Design review of the part built by this model. Coordinates are the model's own, in mm. A direction names the side the tool comes from. Coordinates: 2 decimals unless noted, no trailing zeros. Write each loop counter-clockwise with the first axis right and the second up, starting at its lowest first coordinate (ties: lowest second). Pieces come first, ordered by that corner, then holes.
Q1. Mouldability with a two-part tool opening along Z and no side actions: class faces 1 (the flat face through (6.324, 7.395, -27.347)), 2 (the flat face through (-5.32, 32.96, 32.43)), 3 (the flat face through (-9, 7, -16)), 4 (the cylindrical face through (-16.545, 7.395, -0.389)) as pulls with the +Z half, pulls with the -Z half, needs draft (parallel to the pull), parting line crosses it, or undercut.
Q2. Take a section at C-C (z = -9). Give the boundary of the cut face in (x, y).
Q3. Take a section at D-D (z = 26). Give the boundary of the cut face in (x, y).
Q4. Insertion check: pin 1 (4 mm diameter, centred on y = 6, z = -16.5, fed in from +X); pin 2 (3 mm diameter, centred on y = 27, z = 35.5, fed in from -X); pin 3 (1.2 mm diameter, centred on x = -7.5, y = 33, fed in from -Z); pin 4 (1.5 mm diameter, centred on x = -10, z = 10, fed in from -Y). Each pin has a flat end and moves straight along its axis. Give the tip position at first contact, or say it passes through.
Q5. For probe 1 along Z at (x, y) = (9.5, 4.5); probe 2 along Z at (x, y) = (-9.5, 22); probe 3 along Z at (x, y) = (8, 16.5), list the stretches that pass through material, from the lowest coordinate up.
Q6. Machinability: for faces 5 (the flat face through (9, 33, 31.469)), 6 (the flat face through (5, 7, -17.756)), 7 (the flat face through (10, 32, 35)), 8 (the flat face through (-10, 25, 20)), 9 (the flat face through (-9, 33, 31.469)), which of the approach directions +Z, -Z, +X, -X, +Y, -Y give a long, thin tool a straight path to every point of the face, cutting with its end or side? Answer none if there is none.
Q7. Take a section at B-B (y = 28.5). Give the boundary of the cut face in (x, z), and give its area (3 significant figures).
Q8. Take a section at A-A (x = -11.5). Give the boundary of the cut face in (y, z), and give its area (3 significant figures).
Autodesk Inventor part; units mm, degrees
ref_plane "YZ Plane" through (0, 0, 0) normal (1, 0, 0) x (0, 1, 0)
ref_plane "XZ Plane" through (0, 0, 0) normal (0, 1, 0) x (-1, 0, 0)
ref_plane "XY Plane" through (0, 0, 0) normal (0, 0, 1) x (1, 0, 0)
sketch "스케치1" plane through (0, 0, 0) normal (0, 1, 0) x (-1, 0, 0)
  arc A0 (0, -14.55) -> (-2.5266, -14.329) centre (0, 0) ccw
  line L0 (-2.5656, -14.55) -> (-7, -14.55)
  line L1 (7, -14.55) -> (7, -12.7555)
  line L2 (-7, -14.55) -> (-7, -12.7555)
  arc A1 (2.8739, -16.2986) -> (-2.8739, -16.2986) centre (0, 0) ccw
  line L3 (7, -12.7555) -> (7, -17.7555)
  line L4 (-7, -12.7555) -> (-7, -17.7555)
  line L5 (-7, -17.7555) -> (-9, -17.7555)
  line L6 (-9, -17.7555) -> (-9, -13.8889)
  line L7 (7, -17.7555) -> (9, -17.7555)
  line L8 (9, -17.7555) -> (9, -13.8889)
  line L9 (0, 0) -> (23.7529, 0) construction
  line L10 (0, 0) -> (23.7529, 0) construction
  line L11 (4.1247, -23.3921) -> (7.0791, -22.8711)
  line L12 (7.0791, -22.8711) -> (6.1771, -17.7555)
  line L13 (-4.1247, -23.3921) -> (-7.0791, -22.8711)
  line L14 (-7.0791, -22.8711) -> (-6.1771, -17.7555)
  line L15 (-7, -17.7555) -> (-3.1308, -17.7555)
  line L16 (-9, -17.7555) -> (-9, -18.7555)
  line L17 (-9, -18.7555) -> (-6.3534, -18.7555)
  line L18 (9, -17.7555) -> (9, -18.7555)
  line L19 (9, -18.7555) -> (6.3534, -18.7555)
  line L20 (7, -17.7555) -> (6.1771, -17.7555)
  line L21 (6.1771, -17.7555) -> (3.1308, -17.7555)
  line L22 (0, 0) -> (-2.8739, -16.2986)
  line L23 (-3.1308, -17.7555) -> (-4.1247, -23.3921)
  line L24 (0, 0) -> (2.8739, -16.2986)
  line L25 (3.1308, -17.7555) -> (4.1247, -23.3921)
  line L26 (-7, -14.55) -> (-2.5656, -14.55)
  line L27 (0, -14.55) -> (7, -14.55)
  line L28 (3.1308, -17.7555) -> (4.8673, -27.6036)
  line L29 (4.8673, -27.6036) -> (7.8217, -27.0826)
  line L30 (7.8217, -27.0826) -> (7.0791, -22.8711)
  line L31 (-3.1308, -17.7555) -> (-4.8673, -27.6036)
  line L32 (-4.8673, -27.6036) -> (-7.8217, -27.0826)
  line L33 (-7.8217, -27.0826) -> (-7.0791, -22.8711)
  point P0 (-7, -14.9967)
  dimension "d0" = 29.1
  dimension "d1" = 7
  dimension "d2" = 14
  dimension "d3" = 2
  dimension "d4" = 5
  dimension "d5" = 2
  dimension "d6" = 2
  dimension "d7" = 5
  dimension "d10" = 3
  dimension "d11" = 1
  dimension "d14" = 10
  dimension "d15" = 10
extrude "돌출1" add sketch "스케치1" along normal blind 15 contours A0 L2 L4 A1 L3 L1 | A1 L8 L7 L3 | L4 L5 L6 A1 | L7 L18 L19 L12 L20 | L15 L14 L17 L16 L5 | L12 L11 L25 L21 | L15 L23 L13 L14 | L30 L29 L28 L11 | L13 L31 L32 L33
sketch "스케치2" plane through (7.8217, 0, -27.0826) normal (0.9848, 0, 0.1736) x (0.1736, 0, -0.9848)
  line L0 (0, 0) -> (0, 15)
  line L1 (-8.4556, 0) -> (-8.4556, 15)
  line L2 (0, 15) -> (-8.4556, 15)
  circle A0 centre (-4.2278, 7.5) radius 2.1
  point P0 (-28.0294, 0)
  dimension "d16" = 4.2
extrude "돌출2" cut sketch "스케치2" against normal up to surface (3 mm away)
sketch "스케치3" plane through (-6.3534, 0, -18.7555) normal (-0.9848, 0, 0.1736) x (0.1736, 0, 0.9848)
  line L0 (1.5444, 0) -> (-8.4556, 0)
  line L1 (0, 0) -> (0, 15)
  line L2 (-8.4556, 0) -> (0, 0)
  circle A0 centre (-4.2278, 7.5) radius 2.1
  point P0 (19.5738, 0)
  dimension "d19" = 4.2
extrude "돌출3" cut sketch "스케치3" against normal up to surface (3 mm away)
sketch "스케치4" plane through (0, 15, 0) normal (0, 1, 0) x (1, 0, 0)
  circle A0 centre (0, 0) radius 16.55
  line L0 (-10, -22.55) -> (10, -22.55)
  line L1 (10, -22.55) -> (10, -10.55)
  line L2 (10, -10.55) -> (-10, -10.55)
  line L3 (-10, -10.55) -> (-10, -22.55)
  arc A1 (-9, 13.8889) -> (9, 13.8889) centre (0, 0) ccw
  line L4 (-10, -22.55) -> (10, -10.55) construction
  line L5 (10, -22.55) -> (-10, -10.55) construction
  point P0 (0, -16.55)
  point P1 (10, -13.1872)
  point P2 (-10, -13.1872)
  dimension "d22" = 20
  dimension "d23" = 12
extrude "돌출4" add sketch "스케치4" against normal up to surface (15 mm away) contours L1 L0 L3 A0
sketch "스케치5" plane through (0, 15, 0) normal (0, 1, 0) x (1, 0, 0)
  line L0 (-10, -13.1872) -> (-10, -22.55)
  line L1 (-10, -17.8686) -> (10, -17.8686)
  line L2 (10, -17.8686) -> (10, -37.8686)
  line L3 (10, -37.8686) -> (-10, -37.8686)
  line L4 (-10, -37.8686) -> (-10, -17.8686)
  point P0 (0, 0)
  dimension "d26" = 20
  dimension "d27" = 20
extrude "돌출5" add sketch "스케치5" along normal blind 50 and the other way blind 15
sketch "스케치6" plane through (0, 65, 0) normal (0, 1, 0) x (1, 0, 0)
  line L0 (-10, -13.1872) -> (-10, -17.8686)
  line L1 (-10, -37.8686) -> (-10, -13.1872)
  line L2 (-10, -17.8686) -> (-10, -37.8686)
  line L3 (-10, -37.8686) -> (-10, -27.8686)
  line L4 (-10, -27.8686) -> (-10, -24.7686)
  line L5 (-10, -27.8686) -> (-10, -24.2686)
  line L6 (-10, -27.8686) -> (-10, -22.3686)
  line L7 (-10, -24.2686) -> (-8.2, -24.2686)
  line L8 (-8.2, -24.2686) -> (-8.2, -22.3686)
  line L9 (-8.2, -22.3686) -> (-6.7, -22.3686)
  line L10 (-10, -22.3686) -> (-3.9, -22.3686)
  line L11 (-6.7, -22.3686) -> (-3.9, -24.2686)
  line L12 (-3.9, -24.2686) -> (-3.9, -27.8686)
  line L13 (-10, -27.8686) -> (-3.9, -27.8686)
  line L14 (-10, -31.4686) -> (-8.2, -31.4686)
  line L15 (-8.2, -31.4686) -> (-8.2, -33.3686)
  line L16 (-8.2, -33.3686) -> (-6.7, -33.3686)
  line L17 (-6.7, -33.3686) -> (-3.9, -31.4686)
  line L18 (-3.9, -31.4686) -> (-3.9, -27.8686)
  line L19 (-10, -27.8686) -> (-10, -17.8686)
  point P0 (0, 0)
  point P1 (-10, -31.4686)
  dimension "d32" = 3.1
  dimension "d33" = 3.6
  dimension "d34" = 5.5
  dimension "d35" = 1.8
  dimension "d36" = 1.5
  dimension "d37" = 6.1
  dimension "d40" = 10
extrude "돌출6" cut sketch "스케치6" against normal through all contours L1 L13 L18 L17 L16 L15 L14 | L1 L7 L8 L9 L11 L12 L13
mirror "미러1" about plane through (0, 0, 0) normal (1, 0, 0) of "돌출6"
properties part number "USB_camera"
Response:
1. face 1: pulls with the -Z half
1. face 2: undercut
1. face 3: needs draft
1. face 4: parting line crosses it
2. outline: (-13.89, 0) - (-11.43, 0) - (-11.43, 15) - (-13.89, 15) - close; (11.43, 0) - (13.89, 0) - (13.89, 15) - (11.43, 15) - close
3. outline: (-3.9, 0) - (3.9, 0) - (3.9, 65) - (-3.9, 65) - close
4. pin 1: stops at x = 9
4. pin 2: stops at x = -10
4. pin 3: stops at z = 17.87
4. pin 4: stops at y = 0
5. probe 1: z = -13.55 to -11.02, 11.02 to 24.27, 31.47 to 37.87
5. probe 2: z = 17.87 to 24.27, 31.47 to 37.87
5. probe 3: z = 17.87 to 22.37, 33.37 to 37.87
6. face 5: +X, +Y, -Y
6. face 6: +Y, -Y
6. face 7: +Z, +X, +Y, -Y
6. face 8: +Z, -X, +Y, -Y
6. face 9: -X, +Y, -Y
7. outline: (-10, 17.87) - (10, 17.87) - (10, 24.27) - (8.2, 24.27) - (8.2, 22.37) - (6.7, 22.37) - (3.9, 24.27) - (3.9, 31.47) - (6.7, 33.37) - (8.2, 33.37) - (8.2, 31.47) - (10, 31.47) - (10, 37.87) - (-10, 37.87) - (-10, 31.47) - (-8.2, 31.47) - (-8.2, 33.37) - (-6.7, 33.37) - (-3.9, 31.47) - (-3.9, 24.27) - (-6.7, 22.37) - (-8.2, 22.37) - (-8.2, 24.27) - (-10, 24.27) - close
7. area: 290 mm2
8. outline: (0, -11.9) - (15, -11.9) - (15, -8.91) - (0, -8.91) - close; (0, 8.91) - (15, 8.91) - (15, 11.9) - (0, 11.9) - close
8. area: 89.7 mm2
